Could you check a few things on this model? Use its own coordinates, in mm. Face numbers are marked on the shaded views. A direction names the side the tool comes from. Give positions to 0.01 mm unless a question says otherwise; leave off trailing zeros. Order: outer loops, then holes, each group sorted by start corner. A loop starts at its lowest first (then second) coordinate and runs counter-clockwise, first axis right, second up. Notation, with made-up numbers: (32.5, 86.5) -> (87.5, 86.5) arc R10 cw to (87.5, 105.5) -> close; hole circle Ø2 at (89.25, 62). An arc over 180 degrees is marked (long way). Answer as CSV lines item,"result". Start each with the question number.
(1) Will these pins go through, and if not, where does the flat tip stop? pin 1 Ø1.2 at (y, z) = (4.5, -14.5) entering from -X; pin 2 Ø1.5 at (x, z) = (4.5, -10.5) entering from +Y; pin 3 Ø6.5 at (y, z) = (19.5, -10) entering from +X.
(2) I want a section at B-B (y = 14). Please give me the cut outline in (x, z), plus the area to 3 significant figures.
(3) We'd pull the mould along X, two halves only. Please class the marked faces 1, 2, 3 and 4: released by +X, released by -X, zero draft, split by the parting line, or undercut.
(4) I need wall thicknesses on L1, parallel to Z at x = -8.75, y = 21; L2, parallel to X at y = 14.5, z = -10.75; L3, parallel to Y at x = -8, z = -2.25. Which ranges of each line are inside material? Lowest first, please.
(5) I want a section at C-C (z = -10). Give the number of separate pieces and of enclosed holes in the cut face, plus the area to 3 significant figures.
(6) On a 3-axis mill with a long thin cutter (end or side, diameter ignored), from which of +Z, -Z, +X, -X, +Y, -Y can I reach the whole of each face in a straight line? I mean the marked faces 5, 6 and 7. Say none if no direction works.
(7) I want a section at A-A (y = 17.5). Please give me the cut outline in (x, z).
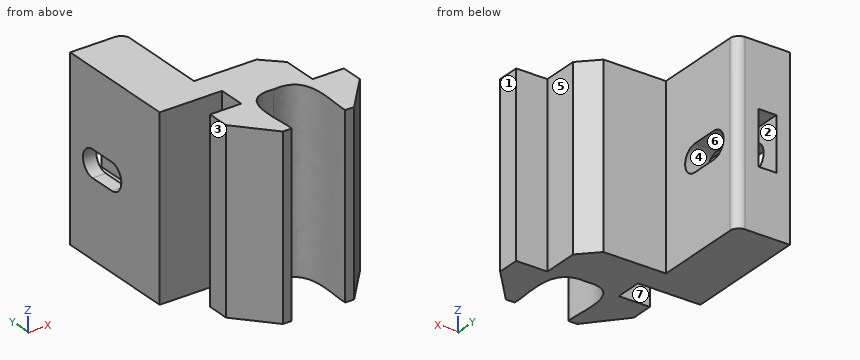
```python
from build123d import *

# Parameters (mm, degrees)
ESTRUSIONE_ESTRUSIONE1_DEPTH  = 20
TAGLIO_ESTRUSIONE1_REACH      = 37.979
SCHIZZO12_W                   = 2
SCHIZZO12_H                   = 6
TAGLIO_ESTRUSIONE2_DEPTH      = 11
TAGLIO_ESTRUSIONE3_DEPTH      = 33.760494502
TAGLIO_ESTRUSIONE3_DEPTH_BACK = 33.760494502
SMUSSO1_SIZE                  = 2


with BuildPart() as part:
    # Schizzo2 → Estrusione-Estrusione1 (new body)
    with BuildSketch(Plane.XY):
        with BuildLine():
            Line((-4, 9.5), (-11, 9.5))
            Line((-11, 9.5), (-11, 23.5))
            Line((-11, 23.5), (-6, 23.5))
            ThreePointArc((-6, 23.5), (-5.292893219, 23.207106781), (-5, 22.5))
            Line((-5, 22.5), (-5, 12.5))
            Line((-5, 12.5), (4, 12.5))
            Line((4, 12.5), (4, 9.5))
            Line((4, 9.5), (4, 6.5))
            Line((4, 6.5), (7.5, 6.5))
            Line((7.5, 6.5), (7.5, 4))
            Line((7.5, 4), (4, 0))
            Line((4, 0), (-4, 0))
            Line((-4, 0), (-7.5, 4))
            Line((-7.5, 4), (-7.5, 6.5))
            Line((-7.5, 6.5), (-4, 6.5))
            Line((-4, 6.5), (-4, 9.5))
        make_face()
    extrude(amount=-ESTRUSIONE_ESTRUSIONE1_DEPTH)

    # Schizzo6 → Taglio-Estrusione1 (cut, up to next)
    with BuildSketch(Plane.ZY.offset(11), mode=Mode.PRIVATE) as taglio_estrusione1_sk1:
        with BuildLine():
            Line((-8.5, 20), (-8.5, 17))
            ThreePointArc((-8.5, 17), (-10, 15.5), (-11.5, 17))
            Line((-11.5, 17), (-11.5, 20))
            ThreePointArc((-11.5, 20), (-10, 21.5), (-8.5, 20))
        make_face()
    taglio_estrusione1_tool1 = extrude(taglio_estrusione1_sk1.sketch, amount=-TAGLIO_ESTRUSIONE1_REACH, mode=Mode.PRIVATE) & part.part
    add(taglio_estrusione1_tool1.solids().sort_by_distance((-11, 18.5, -10))[0], mode=Mode.SUBTRACT)

    # Schizzo12 → Taglio-Estrusione2 (cut)
    with BuildSketch(Plane(origin=(0, 23.5, 0), x_dir=(1, 0, 0), z_dir=(0, 1, 0))):
        with Locations((-8.5, 10)):
            Rectangle(SCHIZZO12_W, SCHIZZO12_H)
    extrude(amount=-TAGLIO_ESTRUSIONE2_DEPTH, mode=Mode.SUBTRACT)

    # Schizzo13 → Taglio-Estrusione3 (cut, two sides: drawn at the far end of the back side and taken through both)
    with BuildSketch(Plane(origin=(0, 0, -20), x_dir=(-1, 0, 0), z_dir=(0, 0, -1)).offset(-TAGLIO_ESTRUSIONE3_DEPTH_BACK)):
        with BuildLine():
            add(Edge.make_bspline(
                [(-3, 0), (-2.831721027, 2.145011642), (-4.377617752, 7.500745545), (0, 7)],
                knots=[0, 0, 0, 0, 1, 1, 1, 1], degree=3))
            Line((-3, 0), (3, 0))
            add(Edge.make_bspline(
                [(3, 0), (2.831721027, 2.145011642), (4.377617752, 7.500745545), (0, 7)],
                knots=[0, 0, 0, 0, 1, 1, 1, 1], degree=3))
        make_face()
    extrude(amount=TAGLIO_ESTRUSIONE3_DEPTH + TAGLIO_ESTRUSIONE3_DEPTH_BACK, mode=Mode.SUBTRACT)

    # Smusso1
    smusso1_edges = [part.edges().sort_by_distance(p)[0] for p in [
        (4, 12.5, -10),
    ]]
    chamfer(smusso1_edges, length=SMUSSO1_SIZE)


solid = part.part
```
Final values:
1,pin 1,"x = -7.5"
1,pin 2,"y = 10.75"
1,pin 3,"x = -5"
2,outline,"(-11, -20) -> (-5, -20) -> (-5, 0) -> (-11, 0) -> close; hole (-9.5, -13) -> (-7.5, -13) -> (-7.5, -7) -> (-9.5, -7) -> close"
2,area,"108 mm²"
3,face 1,"released by +X"
3,face 2,"undercut"
3,face 3,"released by -X"
3,face 4,"zero draft"
4,L1,"-20 to -13, -7 to 0"
4,L2,"-11 to -9.5, -7.5 to -5"
4,L3,"9.5 to 23.5"
5,separate pieces,"3"
5,enclosed holes,"0"
5,area,"130 mm²"
6,face 5,"+Z, -Z, +X, +Y"
6,face 6,"+X, -X"
6,face 7,"+Z, -Z, -X"
7,outline,"(-11, -20) -> (-5, -20) -> (-5, -11.5) -> (-7.5, -11.5) -> (-7.5, -13) -> (-9.5, -13) -> (-9.5, -11.5) -> (-11, -11.5) -> close; (-11, -8.5) -> (-9.5, -8.5) -> (-9.5, -7) -> (-7.5, -7) -> (-7.5, -8.5) -> (-5, -8.5) -> (-5, 0) -> (-11, 0) -> close"
